from build123d import *

# Parameters (mm, degrees)
CYLINDER231_R          = 1.4
CYLINDER231_DEPTH      = 20
CYLINDER231_ROLL_ANGLE = 90
CYLINDER230_R          = 1.4
CYLINDER230_DEPTH      = 20
CYLINDER230_ROLL_ANGLE = 90
BOX001027045174_W      = 10
BOX001027045174_H      = 4
BOX001027045174_DEPTH  = 24


with BuildPart() as m3_tap006:
    # Cylinder231 → Cylinder231 (new body)
    with BuildSketch(Plane.XY):
        Circle(CYLINDER231_R)
    extrude(amount=CYLINDER231_DEPTH)


with BuildPart() as m3_tap006_1:
    # Cylinder231 roll: moved
    add(m3_tap006.part.rotate(Axis((0, 0, 0), (1, 0, 0)), CYLINDER231_ROLL_ANGLE))


with BuildPart() as m3_tap006_2:
    # Cylinder231 placement: moved
    add(m3_tap006_1.part.moved(Location((34, 5, -29))))


with BuildPart() as fusion112123:
    # Cylinder230 → Cylinder230 (new body)
    with BuildSketch(Plane.XY):
        Circle(CYLINDER230_R)
    extrude(amount=CYLINDER230_DEPTH)


with BuildPart() as fusion112123_1:
    # Cylinder230 roll: moved
    add(fusion112123.part.rotate(Axis((0, 0, 0), (1, 0, 0)), CYLINDER230_ROLL_ANGLE))


with BuildPart() as fusion112123_2:
    # Cylinder230 placement: moved
    add(fusion112123_1.part.moved(Location((34, 5, -14))))

    # Fusion112123: union M3-tap006
    add(m3_tap006_2.part)


with BuildPart() as join_plate:
    # Box001027045174 → Box001027045174 (new body)
    with BuildSketch(Plane(origin=(29, -8.5, -34), x_dir=(1, 0, 0), z_dir=(0, 0, 1))):
        with Locations((5, 2)):
            Rectangle(BOX001027045174_W, BOX001027045174_H)
    extrude(amount=BOX001027045174_DEPTH)

    # Cut209: cut Fusion112123
    add(fusion112123_2.part, mode=Mode.SUBTRACT)


solid = join_plate.part
Geometry check sheet. Reference: the model listing, model coordinates, mm. Coordinates: 2 decimals unless noted, no trailing zeros. Order: outer loops, then holes, each group sorted by start corner. A loop starts at its lowest first (then second) coordinate and runs counter-clockwise, first axis right, second up. Notation, with made-up numbers: (62, 10.25) - (105, 10.25) arc R13 ccw to (105, 27.25) - close; hole circle Ø4 at (10, 18). An arc over 180 degrees is marked (long way). One line per item, written item: value.
(1) Sectioned sample at A-A (x = 34). Enter the section's corners in (y, z), and give its area (3 significant figures).
Data:
outline: (-8.5, -34) - (-4.5, -34) - (-4.5, -30.4) - (-8.5, -30.4) - close; (-8.5, -27.6) - (-4.5, -27.6) - (-4.5, -15.4) - (-8.5, -15.4) - close; (-8.5, -12.6) - (-4.5, -12.6) - (-4.5, -10) - (-8.5, -10) - close
area: 73.6 mm^2
(2) Thickness scan on probe 1 along Z at (x, y) = (34, -5.8); probe 2 along Z at (x, y) = (33.25, -6.5); probe 3 along X at (y, z) = (-6.9, -29). Record the ranges inside material, lowest first. Write a range as from..to.
Data:
probe 1: z = -34..-30.4, -27.6..-15.4, -12.6..-10
probe 2: z = -34..-30.18, -27.82..-15.18, -12.82..-10
probe 3: x = 29..32.6, 35.4..39
(3) Release check for a two-part mould opening along Z. For faces 1 (the face through (29, -7, -22)), 2 (the face through (34, -6, -10)), 3 (the face through (32.97, -6.47, -13.05)) record: +Z half, -Z half, draft (parallel to the pull), parting line (faces both ways), or undercut.
Data:
face 1: draft
face 2: +Z half
face 3: undercut
(4) Sectioned sample at D-D (z = -13.5). Enter the section's corners in (x, y), and give its area (3 significant figures).
Data:
outline: (29, -8.5) - (32.69, -8.5) - (32.69, -4.5) - (29, -4.5) - close; (35.31, -8.5) - (39, -8.5) - (39, -4.5) - (35.31, -4.5) - close
area: 29.5 mm^2
(5) Depth check by flat-ended pin: pin 1 Ø2.5 at (x, z) = (34, -29) entering from -Y; pin 2 Ø4.5 at (x, z) = (34, -14) entering from -Y. Enter the tip coordinate at first touch or a pass-through.
Data:
pin 1: passes through
pin 2: stops at y = -8.5
(6) Sectioned sample at B-B (z = -29). Enter the section's corners in (x, y), and give its area (3 significant figures).
Data:
outline: (29, -8.5) - (32.6, -8.5) - (32.6, -4.5) - (29, -4.5) - close; (35.4, -8.5) - (39, -8.5) - (39, -4.5) - (35.4, -4.5) - close
area: 28.8 mm^2
(7) Sectioned sample at C-C (y = -4.75). Enter the section's corners in (x, z).
Data:
outline: (29, -34) - (39, -34) - (39, -10) - (29, -10) - close; hole circle Ø2.8 at (34, -29); hole circle Ø2.8 at (34, -14)
